The listing builds one solid part. Answer for the finished solid, in the listing's coordinates (mm). A direction names the side the tool comes from. Coordinates: 2 decimals unless noted, no trailing zeros. Order: outer loops, then holes, each group sorted by start corner. A loop starts at its lowest first (then second) coordinate and runs counter-clockwise, first axis right, second up. Notation, with made-up numbers: (52.5, 31) -> (103.5, 31) arc R15 ccw to (103.5, 52) -> close; hole circle Ø1 at (35.25, 31.5). An arc over 180 degrees is marked (long way). Answer in a Markdown table with one row per item.
```python
from build123d import *

# Parameters (mm, degrees)
F1_DEPTH = 25.4


with BuildPart() as f1:
    # F0 (on Front) → F1 (new body)
    with BuildSketch(Plane.XZ):
        with BuildLine():
            ThreePointArc((-9.428049, 1.355549), (-8.664245, 3.956828), (-7.198515, 6.237548))
            Line((-7.198515, 6.237548), (-27.395362, 16.048571))
            ThreePointArc((-27.395362, 16.048571), (-28.880816, 13.189427), (-30.068848, 10.194454))
            Line((-30.068848, 10.194454), (-9.428049, 1.355549))
        make_face()
        with BuildLine():
            ThreePointArc((-7.198515, 6.237548), (-5.149604, 8.01294), (-2.683503, 9.139171))
            Line((-2.683503, 9.139171), (-14.369933, 28.311968))
            ThreePointArc((-14.369933, 28.311968), (-17.165346, 26.7098), (-19.783986, 24.832567))
            Line((-19.783986, 24.832567), (-7.198515, 6.237548))
        make_face()
        with BuildLine():
            ThreePointArc((9.525, 0), (9.500731, 0.679506), (9.428049, 1.355549))
            ThreePointArc((9.428049, 1.355549), (8.664245, 3.956828), (7.198515, 6.237548))
            ThreePointArc((7.198515, 6.237548), (5.149604, 8.01294), (2.683503, 9.139171))
            ThreePointArc((2.683503, 9.139171), (0, 9.525), (-2.683503, 9.139171))
            ThreePointArc((-2.683503, 9.139171), (-5.149604, 8.01294), (-7.198515, 6.237548))
            ThreePointArc((-7.198515, 6.237548), (-8.664245, 3.956828), (-9.428049, 1.355549))
            ThreePointArc((-9.428049, 1.355549), (-9.428049, -1.355549), (-8.664245, -3.956828))
            ThreePointArc((-8.664245, -3.956828), (-7.198515, -6.237548), (-5.149604, -8.01294))
            ThreePointArc((-5.149604, -8.01294), (-2.683503, -9.139171), (0, -9.525))
            ThreePointArc((0, -9.525), (2.683503, -9.139171), (5.149604, -8.01294))
            ThreePointArc((5.149604, -8.01294), (7.198515, -6.237548), (8.664245, -3.956828))
            ThreePointArc((8.664245, -3.956828), (9.307324, -2.024684), (9.525, 0))
        make_face()
        with BuildLine():
            ThreePointArc((3.175, 0), (2.245064, -2.245064), (0, -3.175))
            ThreePointArc((0, -3.175), (-2.245064, 2.245064), (3.175, 0))
        make_face(mode=Mode.SUBTRACT)
        with BuildLine():
            ThreePointArc((-2.683503, 9.139171), (0, 9.525), (2.683503, 9.139171))
            Line((2.683503, 9.139171), (3.217849, 31.586515))
            ThreePointArc((3.217849, 31.586515), (0, 31.75), (-3.217849, 31.586515))
            Line((-3.217849, 31.586515), (-2.683503, 9.139171))
        make_face()
        with BuildLine():
            Line((7.198515, 6.237548), (19.783986, 24.832567))
            ThreePointArc((19.783986, 24.832567), (17.165346, 26.7098), (14.369933, 28.311968))
            Line((14.369933, 28.311968), (2.683503, 9.139171))
            ThreePointArc((2.683503, 9.139171), (5.149604, 8.01294), (7.198515, 6.237548))
        make_face()
        with BuildLine():
            Line((9.428049, 1.355549), (30.068848, 10.194454))
            ThreePointArc((30.068848, 10.194454), (28.880816, 13.189427), (27.395362, 16.048571))
            Line((27.395362, 16.048571), (7.198515, 6.237548))
            ThreePointArc((7.198515, 6.237548), (8.664245, 3.956828), (9.428049, 1.355549))
        make_face()
        with BuildLine():
            ThreePointArc((30.807062, -7.680326), (31.426831, -4.518496), (31.722958, -1.310134))
            Line((31.722958, -1.310134), (9.428049, 1.355549))
            ThreePointArc((9.428049, 1.355549), (9.500731, 0.679506), (9.525, 0))
            ThreePointArc((9.525, 0), (9.307324, -2.024684), (8.664245, -3.956828))
            Line((8.664245, -3.956828), (30.807062, -7.680326))
        make_face()
        with BuildLine():
            ThreePointArc((21.764252, -23.116657), (23.995049, -20.791828), (25.978738, -18.252881))
            Line((25.978738, -18.252881), (8.664245, -3.956828))
            ThreePointArc((8.664245, -3.956828), (7.198515, -6.237548), (5.149604, -8.01294))
            Line((5.149604, -8.01294), (21.764252, -23.116657))
        make_face()
        with BuildLine():
            Line((11.986453, -29.400467), (5.149604, -8.01294))
            ThreePointArc((5.149604, -8.01294), (2.683503, -9.139171), (0, -9.525))
            Line((0, -9.525), (5.811446, -31.213612))
            ThreePointArc((5.811446, -31.213612), (8.945009, -30.463902), (11.986453, -29.400467))
        make_face()
        with BuildLine():
            Line((-5.811446, -31.213612), (0, -9.525))
            ThreePointArc((0, -9.525), (-2.683503, -9.139171), (-5.149604, -8.01294))
            Line((-5.149604, -8.01294), (-11.986453, -29.400467))
            ThreePointArc((-11.986453, -29.400467), (-8.945009, -30.463902), (-5.811446, -31.213612))
        make_face()
        with BuildLine():
            Line((-21.764252, -23.116657), (-5.149604, -8.01294))
            ThreePointArc((-5.149604, -8.01294), (-7.198515, -6.237548), (-8.664245, -3.956828))
            Line((-8.664245, -3.956828), (-25.978738, -18.252881))
            ThreePointArc((-25.978738, -18.252881), (-23.995049, -20.791828), (-21.764252, -23.116657))
        make_face()
        with BuildLine():
            ThreePointArc((-8.664245, -3.956828), (-9.428049, -1.355549), (-9.428049, 1.355549))
            Line((-9.428049, 1.355549), (-31.722958, -1.310134))
            ThreePointArc((-31.722958, -1.310134), (-31.426831, -4.518496), (-30.807062, -7.680326))
            Line((-30.807062, -7.680326), (-8.664245, -3.956828))
        make_face()
    extrude(amount=F1_DEPTH)


solid = f1.part
```
(1) Find the intervals of material crossed by line 1 along Z through (x, y) = (25, -17.25); line 2 along Z through (x, y) = (20.5, -23.5); line 3 along Z through (x, y) = (14.5, -23), in increasing order. Write a range as from..to.
Check values:
| item | result |
|---|---|
| line 1 | -19.57..-17.44, -6.7..-0.51, 8.02..14.88 |
| line 2 | -21.97..-13.73, -5.95..0.03, 6.1..12.7 |
| line 3 | -16.51..-8.78, -4.94..0.75, 3.53..9.78, 17.03..28.25 |
(2) A cutting plane is placed at B-B, the plane z = -12. Determine the outline of the cut face in (x, y).
Check values:
| item | result |
|---|---|
| outline | (-18.41, -25.4) -> (-9.54, -25.4) -> (-9.54, 0) -> (-18.41, 0) -> close; (-6.42, -25.4) -> (-0.66, -25.4) -> (-0.66, 0) -> (-6.42, 0) -> close; (0.66, -25.4) -> (6.42, -25.4) -> (6.42, 0) -> (0.66, 0) -> close; (9.54, -25.4) -> (18.41, -25.4) -> (18.41, 0) -> (9.54, 0) -> close |
(3) Which of the six approach directions +Z, -Z, +X, -X, +Y, -Y give full straight-line access (tool end or side, diameter ignored) to faces 1 (the flat face through (17.443, -12.522, -11.205)), 2 (the flat face through (-2.946, -12.522, -20.521)), 3 (the flat face through (20.732, -12.522, 0.004))?
Check values:
| item | result |
|---|---|
| face 1 | +Y, -Y |
| face 2 | -Z, +Y, -Y |
| face 3 | +X, +Y, -Y |
(4) Flat-ended cylindrical pins translate along their axes: pin 1 (1.5 mm diameter, centred on x = -21.5, y = -17.5, fed in from +Z); pin 2 (2 mm diameter, centred on x = -13.5, y = -10, fed in from +Z); pin 3 (4 mm diameter, centred on x = 7, y = -8.5, fed in from +Z). Find the tip coordinate at first contact, or state that the pin passes through.
Check values:
| item | result |
|---|---|
| pin 1 | z = 13.55 |
| pin 2 | z = 28.31 |
| pin 3 | z = 19.5 |
(5) A cutting plane is placed at A-A, the plane x = -17. Determine the outline of the cut face in (y, z), then the cut area to 3 significant figures.
Check values:
| item | result |
|---|---|
| outline | (-25.4, -18.79) -> (0, -18.79) -> (0, -10.84) -> (-25.4, -10.84) -> close; (-25.4, -5.36) -> (0, -5.36) -> (0, 0.45) -> (-25.4, 0.45) -> close; (-25.4, 4.6) -> (0, 4.6) -> (0, 11) -> (-25.4, 11) -> close; (-25.4, 20.72) -> (0, 20.72) -> (0, 26.82) -> (-25.4, 26.82) -> close |
| area | 667 mm² |
(6) For a pull along Z with two mould halves and no side action, classify faces 4 (the cylindrical face through (28.9, -12.52, 13.15)), 5 (the flat face through (8.616, -12.522, -18.856)), 6 (the cylindrical face through (-24.02, -12.52, -20.76)), 7 (the flat face through (7, -25.4, 1)) as released by +Z, released by -Z, zero draft, split by the parting line, or undercut.
Check values:
| item | result |
|---|---|
| face 4 | released by +Z |
| face 5 | undercut |
| face 6 | released by -Z |
| face 7 | zero draft |
